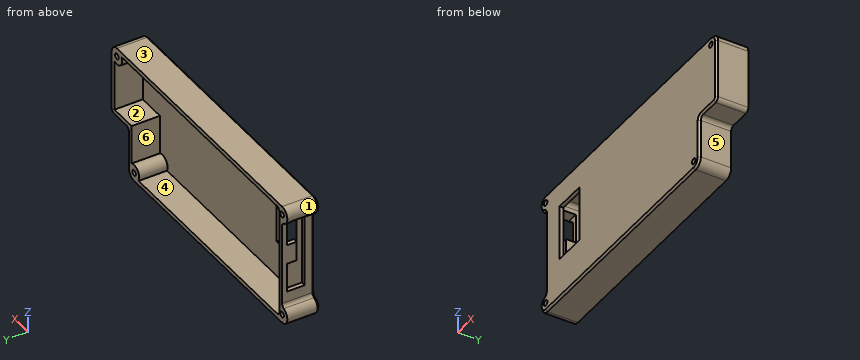
from build123d import *

# Parameters (mm, degrees)
BOSS_EXTRUDE1_DEPTH            = 16.5
BOSS_EXTRUDE2_DEPTH            = 2
FILLET6_R                      = 2
FILLET8_R                      = 2
BOSS_EXTRUDE6_DEPTH            = 16.5
F_2_9_2_9_DIAMETER_HOLE2_D     = 2.9
F_2_9_2_9_DIAMETER_HOLE1_D     = 2.9
SKETCH24_R                     = 4.3
BOSS_EXTRUDE7_DEPTH            = 14.5
F_2_9_2_9_DIAMETER_HOLE3_D     = 2.9
F_2_9_2_9_DIAMETER_HOLE4_D     = 2.9
FILLET10_R                     = 4.3
FILLET16_R                     = 4.3
FILLET17_R                     = 2
FILLET18_R                     = 2
CHAMFER5_SIZE                  = 1
SKETCH29_W                     = 16.5
SKETCH29_H                     = 28.5
CUT_EXTRUDE1_DEPTH             = 10
CUT_EXTRUDE2_REACH             = 148.941
SKETCH30_W                     = 10
SKETCH30_H                     = 4.042033075
SKETCH30_W_2                   = 3.474110813
SKETCH30_H_2                   = 9
CUT_EXTRUDE2_DIRECTION_2_DEPTH = 147.941105233


with BuildPart() as part:
    # Sketch3 → Boss-Extrude1 (new body)
    with BuildSketch(Plane(origin=(0, 0, 0), x_dir=(1, 0, 0), z_dir=(0, 1, 0))):
        Polygon((52.738233838, 8.405993834), (67.038233838, 8.405993834), (67.038233838, -28.194006166), (52.738233838, -28.194006166), (-74.861766162, -28.194006166), (-74.861766162, 34.405993834), (52.738233838, 34.405993834), align=None)
        Polygon((55.038233838, -25.894006166), (64.738233838, -25.894006166), (64.738233838, 6.105993834), (50.438233838, 6.105993834), (50.438233838, 32.105993834), (-72.561766162, 32.105993834), (-72.561766162, -25.894006166), (50.438233838, -25.894006166), align=None, mode=Mode.SUBTRACT)
    extrude(amount=BOSS_EXTRUDE1_DEPTH)

    # Sketch5 → Boss-Extrude2 (add)
    with BuildSketch(Plane(origin=(0, 0, 0), x_dir=(1, 0, 0), z_dir=(0, 1, 0))):
        Polygon((-72.561766162, 32.105993834), (50.438233838, 32.105993834), (50.438233838, 6.105993834), (64.738233838, 6.105993834), (64.738233838, -25.894006166), (50.438233838, -25.894006166), (-72.561766162, -25.894006166), align=None)
    extrude(amount=BOSS_EXTRUDE2_DEPTH)

    # Fillet6
    fillet6_edges = [part.edges().sort_by_distance(p)[0] for p in [
        (50.438233838, 9.25, -32.105993834),
    ]]
    fillet(fillet6_edges, radius=FILLET6_R)

    # Fillet8
    fillet8_edges = [part.edges().sort_by_distance(p)[0] for p in [
        (-72.561766162, 9.25, -32.105993834),
        (-72.561766162, 9.25, 25.894006166),
    ]]
    fillet(fillet8_edges, radius=FILLET8_R)

    # Sketch17 → Boss-Extrude6 (add)
    with BuildSketch(Plane(origin=(0, 0, 0), x_dir=(1, 0, 0), z_dir=(0, 1, 0))):
        with BuildLine():
            Line((-74.861766162, 34.405993834), (-74.861766162, 25.805993834))
            ThreePointArc((-74.861766162, 25.805993834), (-79.161766162, 30.105993834), (-74.861766162, 34.405993834))
        make_face()
        with BuildLine():
            Line((-74.861766162, -19.594006166), (-74.861766162, -28.194006166))
            ThreePointArc((-74.861766162, -28.194006166), (-79.161766162, -23.894006166), (-74.861766162, -19.594006166))
        make_face()
    extrude(amount=BOSS_EXTRUDE6_DEPTH)

    # Ø2.9 (2.9) Diameter Hole2 (through all)
    with Locations(Plane(origin=(0, 16.5, 0), x_dir=(1, 0, 0), z_dir=(0, 1, 0))):
        with Locations((-74.861766162, 30.105993834)):
            Hole(F_2_9_2_9_DIAMETER_HOLE2_D / 2)

    # Ø2.9 (2.9) Diameter Hole1 (through all)
    with Locations(Plane(origin=(0, 16.5, 0), x_dir=(1, 0, 0), z_dir=(0, 1, 0))):
        with Locations((-74.861766162, -23.894006166)):
            Hole(F_2_9_2_9_DIAMETER_HOLE1_D / 2)

    # Sketch24 → Boss-Extrude7 (add)
    with BuildSketch(Plane(origin=(0, 2, 0), x_dir=(1, 0, 0), z_dir=(0, 1, 0))):
        with Locations((62.738431143, -23.885848487)):
            Circle(SKETCH24_R)
        with Locations((48.418494527, 30.105993834)):
            Circle(SKETCH24_R)
    extrude(amount=BOSS_EXTRUDE7_DEPTH)

    # Ø2.9 (2.9) Diameter Hole3 (through all)
    with Locations(Plane(origin=(0, 16.5, 0), x_dir=(1, 0, 0), z_dir=(0, 1, 0))):
        with Locations((62.738431143, -23.885848487)):
            Hole(F_2_9_2_9_DIAMETER_HOLE3_D / 2)

    # Ø2.9 (2.9) Diameter Hole4 (through all)
    with Locations(Plane(origin=(0, 16.5, 0), x_dir=(1, 0, 0), z_dir=(0, 1, 0))):
        with Locations((48.418494527, 30.105993834)):
            Hole(F_2_9_2_9_DIAMETER_HOLE4_D / 2)

    # Fillet10
    fillet10_edges = [part.edges().sort_by_distance(p)[0] for p in [
        (52.738233838, 8.25, -34.405993834),
    ]]
    fillet(fillet10_edges, radius=FILLET10_R)

    # Fillet16
    # the kernel refuses this fillet: 4.3 mm, written as the material it takes off along each edge
    with BuildSketch(Plane(origin=(67.038233838, -10.75, 28.194006166), x_dir=(0, 0, -1), z_dir=(0, 1, 0))) as fillet16_piece_1:
        with BuildLine():
            CenterArc((FILLET16_R, FILLET16_R), FILLET16_R, 180, 90)
            Line((0, FILLET16_R), (0, 0))
            Line((0, 0), (FILLET16_R, 0))
        make_face()
    extrude(amount=38, mode=Mode.SUBTRACT)

    # Fillet17
    fillet17_edges = [part.edges().sort_by_distance(p)[0] for p in [
        (52.738233838, 8.25, -8.405993834),
        (67.038233838, 8.25, -8.405993834),
    ]]
    fillet(fillet17_edges, radius=FILLET17_R)

    # Fillet18
    fillet18_edges = [part.edges().sort_by_distance(p)[0] for p in [
        (-74.861766162, 8.25, -25.805993834),
        (-74.861766162, 8.25, 19.594006166),
    ]]
    fillet(fillet18_edges, radius=FILLET18_R)

    # Chamfer5
    chamfer5_edges = [part.edges().sort_by_distance(p)[0] for p in [
        (-13.211766162, 0, -34.405993834),
        (51.478792997, 0, -33.146552993),
        (67.038233838, 0, 8.744006166),
        (65.778792997, 0, 26.934565325),
        (52.738233838, 0, -20.255993834),
        (59.888233838, 0, -8.405993834),
        (66.4524474, 0, -7.820207397),
        (53.324020275, 0, -8.991780272),
        (-79.105793795, 0, 24.585547524),
        (-74.861766162, 0, -3.105993834),
        (-75.2385223, 0, 19.088261462),
        (-75.2385223, 0, -25.300249131),
        (-6.061766162, 0, 28.194006166),
        (-79.105793795, 0, -30.797535193),
    ]]
    chamfer(chamfer5_edges, length=CHAMFER5_SIZE)

    # Sketch29 → Cut-Extrude1 (cut)
    with BuildSketch(Plane(origin=(0, 2, 0), x_dir=(1, 0, 0), z_dir=(0, 1, 0))):
        with Locations((-55.053624673, -0.644006166)):
            Rectangle(SKETCH29_W, SKETCH29_H)
    extrude(amount=-CUT_EXTRUDE1_DEPTH, mode=Mode.SUBTRACT)

    # Sketch30 → Cut-Extrude2 (cut, up to next)
    with BuildSketch(Plane.ZY.offset(74.861766162), mode=Mode.PRIVATE) as cut_extrude2_sk1:
        with Locations((1.394006166, 7.021016538)):
            Rectangle(SKETCH30_W, SKETCH30_H)
    cut_extrude2_tool1 = extrude(cut_extrude2_sk1.sketch, amount=-CUT_EXTRUDE2_REACH, mode=Mode.PRIVATE) & part.part
    # Sketch30 → Cut-Extrude2 (cut, up to next)
    with BuildSketch(Plane.ZY.offset(74.861766162), mode=Mode.PRIVATE) as cut_extrude2_sk2:
        Polygon((-3.605993834, 5), (-3.605993834, 9.042033075), (-3.605993834, 14), (-18.605993834, 14), (-18.605993834, 5), align=None)
    cut_extrude2_tool2 = extrude(cut_extrude2_sk2.sketch, amount=-CUT_EXTRUDE2_REACH, mode=Mode.PRIVATE) & part.part
    # Sketch30 → Cut-Extrude2 (cut, up to next)
    with BuildSketch(Plane.ZY.offset(74.861766162), mode=Mode.PRIVATE) as cut_extrude2_sk3:
        Polygon((6.394006166, 14), (6.394006166, 9.042033075), (6.394006166, 5), (17.919895353, 5), (17.919895353, 14), align=None)
    cut_extrude2_tool3 = extrude(cut_extrude2_sk3.sketch, amount=-CUT_EXTRUDE2_REACH, mode=Mode.PRIVATE) & part.part
    # Sketch30 → Cut-Extrude2 (cut, up to next)
    with BuildSketch(Plane.ZY.offset(74.861766162), mode=Mode.PRIVATE) as cut_extrude2_sk4:
        with Locations((19.656950759, 9.5)):
            Rectangle(SKETCH30_W_2, SKETCH30_H_2)
    cut_extrude2_tool4 = extrude(cut_extrude2_sk4.sketch, amount=-CUT_EXTRUDE2_REACH, mode=Mode.PRIVATE) & part.part
    add(cut_extrude2_tool1.solids().sort_by_distance((-74.861766, 7.021017, 1.394006))[0], mode=Mode.SUBTRACT)
    add(cut_extrude2_tool2.solids().sort_by_distance((-74.861766, 9.5, -11.105994))[0], mode=Mode.SUBTRACT)
    add(cut_extrude2_tool3.solids().sort_by_distance((-74.861766, 9.5, 12.156951))[0], mode=Mode.SUBTRACT)
    add(cut_extrude2_tool4.solids().sort_by_distance((-74.861766, 9.5, 19.656951))[0], mode=Mode.SUBTRACT)

    # Sketch30 → Cut-Extrude2 direction 2 (cut)
    with BuildSketch(Plane.ZY.offset(74.861766162)):
        with Locations((1.394006166, 7.021016538)):
            Rectangle(SKETCH30_W, SKETCH30_H)
        Polygon((-3.605993834, 5), (-3.605993834, 9.042033075), (-3.605993834, 14), (-18.605993834, 14), (-18.605993834, 5), align=None)
        Polygon((6.394006166, 14), (6.394006166, 9.042033075), (6.394006166, 5), (17.919895353, 5), (17.919895353, 14), align=None)
        with Locations((19.656950759, 9.5)):
            Rectangle(SKETCH30_W_2, SKETCH30_H_2)
    extrude(amount=CUT_EXTRUDE2_DIRECTION_2_DEPTH, mode=Mode.SUBTRACT)


solid = part.part
The listing builds one solid part. Answer for the finished solid, in the listing's coordinates (mm). Face numbers are marked on the shaded views. A direction names the side the tool comes from. Round coordinates to 2 decimals unless told otherwise and drop trailing zeros. Write each loop counter-clockwise with the first axis right and the second up, starting at its lowest first coordinate (ties: lowest second). Pieces come first, ordered by that corner, then holes. Notation, with made-up numbers: M -6,73.5 L 52,73.5 A20 ccw 52,94.5 Z; hole C 34,45.25 d11. An arc over 180 degrees is marked long. Write each question's results on one line, items separated by ' | '. Start each with the question number.
Item 1: Given pin 1 Ø1 at (y, z) = (11.5, -28) entering from +X; pin 2 Ø7 at (y, z) = (6, 13) entering from -X; pin 3 Ø1.7 at (x, z) = (-75, 14.5) entering from -Y, each flat-ended and moving along its own axis, determine where each tip first touches the part or whether it passes through.
Item 2: Straight lines are drawn through the part: probe 1 along Z at (x, y) = (-38.5, 8); probe 2 along X at (y, z) = (2.5, 5); probe 3 along Z at (x, y) = (55.5, 4). For each, find the intervals that lie inside material, in ascending order.
Item 3: Find section A-A on z = 8.5. Write down the section's boundary in (x, y).
Item 4: Find section C-C on x = -18.5. Write down the section's boundary in (y, z), and give its area (3 significant figures).
Item 5: Which of the six approach directions +Z, -Z, +X, -X, +Y, -Y give full straight-line access (tool end or side, diameter ignored) to the marked faces 1 and 2?
Item 6: Find section B-B on x = -60. Write down the section's boundary in (y, z), and give its area (3 significant figures).
Item 7: The mould has two halves that part along X. Classify the marked faces 3, 4, 5 and 6: +X half, -X half, draft (parallel to the pull), parting line (faces both ways), or undercut.
Item 8: Find section D-D on y = 7. Give the number of separate pieces and of enclosed holes in the cut face, and give its area (3 significant figures).
Answer block:
1) pin 1: stops at x = 52.74 | pin 2: stops at x = -74.86 | pin 3: stops at y = 0.29
2) probe 1: z = -34.41 to -32.11, 25.89 to 28.19 | probe 2: x = -74.86 to -72.56, 64.74 to 67.04 | probe 3: z = -8.41 to -6.11, 25.89 to 28.19
3) outline: M -74.86,1 L -73.86,0 L -63.3,0 L -63.3,2 L -72.56,2 L -72.56,5 L -74.86,5 Z; M -74.86,14 L -72.56,14 L -72.56,16.5 L -74.86,16.5 Z; M -46.8,0 L 66.04,0 L 67.04,1 L 67.04,16.5 L 64.74,16.5 L 64.74,2 L -46.8,2 Z
4) outline: M 0,-33.41 L 1,-34.41 L 16.5,-34.41 L 16.5,-32.11 L 2,-32.11 L 2,25.89 L 16.5,25.89 L 16.5,28.19 L 1,28.19 L 0,27.19 Z | area: 191 mm²
5) face 1: -X, +Y, -Y | face 2: +Y
6) outline: M 0,-33.41 L 1,-34.41 L 16.5,-34.41 L 16.5,-32.11 L 2,-32.11 L 2,-13.61 L 0,-13.61 Z; M 0,14.89 L 2,14.89 L 2,25.89 L 16.5,25.89 L 16.5,28.19 L 1,28.19 L 0,27.19 Z | area: 134 mm²
7) face 3: draft | face 4: undercut | face 5: +X half | face 6: undercut
8) separate pieces: 1 | enclosed holes: 4 | area: 919 mm²
